Read the model definition and answer for the solid it produces. Units are mm, in the model's axes. A direction names the side the tool comes from. Coordinates: 2 decimals unless noted, no trailing zeros. Order: outer loops, then holes, each group sorted by start corner. A loop starts at its lowest first (then second) coordinate and runs counter-clockwise, first axis right, second up. Notation, with made-up numbers: M 13,30.25 L 67,30.25 A20 ccw 67,53.25 Z; hole C 69.5,38.25 d1. An arc over 180 degrees is marked long. Use a Markdown table: item, result. Add a question column.
1) Each of these flat-tipped pins is pushed along its axis until it touches: pin 1 Ø6 at (x, z) = (-11.5, 4) entering from +Y; pin 2 Ø3 at (x, z) = (-2.5, 0.5) entering from +Y; pin 3 Ø2 at (x, y) = (3, 1.5) entering from +Z; pin 4 Ø2 at (x, z) = (0, -1.5) entering from +Y. Where does it stop, or does it pass through?
2) For faces 1 (the face through (0, 1, 3)), 2 (the face through (-15.5, 1, 0.1)), 3 (the face through (-0.18, 1.4, 1.57)), determine the directions among +Z, -Z, +X, -X, +Y, -Y from which every point of the face is accessible in a straight line to the end or side of a thin tool.
3) The mould has two halves that part along Z. Classify faces 4 (the face through (0.2, 0, 3.4)), 5 (the face through (0.18, -1.4, 1.57)), 6 (the face through (15.5, 1, -0.1)): released by +Z, released by -Z, zero draft, split by the parting line, or undercut.
4) Find section C-C on y = -0.35. Write down the section's boundary in (x, z).
5) Find the intervals of material crossed by probe 1 along X at (y, z) = (0.3, 0.75); probe 2 along Z at (x, y) = (-4, -0.25); probe 3 along Z at (x, y) = (-13.5, 1.3), in increasing order. Write a range as [from, to].
from build123d import *

# Parameters (mm, degrees)
EXTRUDE_THIN1_DEPTH = 2
FILLET1_R           = 2
BOSS_EXTRUDE1_START = 2
BOSS_EXTRUDE1_DEPTH = 2
FILLET2_R           = 2


with BuildPart() as part:
    # Sketch1 → Extrude-Thin1 (new body)
    with BuildSketch(Plane(origin=(0, 0, 0), x_dir=(1, 0, 0), z_dir=(0, 1, 0))):
        with BuildLine():
            Line((12.5, -3), (-12.5, -3))
            ThreePointArc((-12.5, -3), (-15.5, 0), (-12.5, 3))
            Line((-12.5, 3), (12.5, 3))
            ThreePointArc((12.5, 3), (15.5, 0), (12.5, -3))
        make_face()
        with BuildLine():
            Line((12.5, -1), (-12.5, -1))
            ThreePointArc((-12.5, -1), (-13.5, 0), (-12.5, 1))
            Line((-12.5, 1), (12.5, 1))
            ThreePointArc((12.5, 1), (13.5, 0), (12.5, -1))
        make_face(mode=Mode.SUBTRACT)
    extrude(amount=EXTRUDE_THIN1_DEPTH)

    # Fillet1
    fillet1_edges = [part.edges().sort_by_distance(p)[0] for p in [
        (13.5, 2, 0),
        (0, 2, 1),
        (-13.5, 2, 0),
        (0, 2, -1),
    ]]
    fillet(fillet1_edges, radius=FILLET1_R - 0.0001)  # a hair under: the kernel refuses the full size

    # Sketch2 → Boss-Extrude1 (add)
    with BuildSketch(Plane.XZ.offset(BOSS_EXTRUDE1_START)):
        with BuildLine():
            Line((12.5, -5), (-12.5, -5))
            ThreePointArc((-12.5, -5), (-17.5, 0), (-12.5, 5))
            Line((-12.5, 5), (12.5, 5))
            ThreePointArc((12.5, 5), (17.5, 0), (12.5, -5))
        make_face()
        with BuildLine():
            Line((12.5, -1), (-12.5, -1))
            ThreePointArc((-12.5, -1), (-13.5, 0), (-12.5, 1))
            Line((-12.5, 1), (12.5, 1))
            ThreePointArc((12.5, 1), (13.5, 0), (12.5, -1))
        make_face(mode=Mode.SUBTRACT)
    extrude(amount=-BOSS_EXTRUDE1_DEPTH)

    # Fillet2
    fillet2_edges = [part.edges().sort_by_distance(p)[0] for p in [
        (-13.5, -2, 0),
        (0, -2, -1),
        (13.5, -2, 0),
        (0, -2, 1),
        (0, -2, -5),
        (-17.5, -2, 0),
        (0, -2, 5),
        (17.5, -2, 0),
    ]]
    fillet(fillet2_edges, radius=FILLET2_R - 0.0001)  # a hair under: the kernel refuses the full size


solid = part.part
Check result:
| question | item | result |
|---|---|---|
| 1 | pin 1 | stops at y = 2 |
| 1 | pin 2 | stops at y = 1.73 |
| 1 | pin 3 | stops at z = 3 |
| 1 | pin 4 | stops at y = 1.94 |
| 2 | face 1 | +Z, +X, -X, +Y |
| 2 | face 2 | -X, +Y |
| 2 | face 3 | +Y |
| 3 | face 4 | zero draft |
| 3 | face 5 | undercut |
| 3 | face 6 | split by the parting line |
| 4 | outline | M -12.5,-4.97 L 12.5,-4.97 A4.97 ccw 12.5,4.97 L -12.5,4.97 A4.97 ccw Z; hole M -12.5,-1.03 L 12.5,-1.03 A1.03 ccw 12.5,1.03 L -12.5,1.03 A1.03 ccw Z |
| 5 | probe 1 | x = [-15.4, -13.2], [13.2, 15.4] |
| 5 | probe 2 | z = [-4.98, -1.02], [1.02, 4.98] |
| 5 | probe 3 | z = [-2.83, -1.09], [1.09, 2.83] |
